from build123d import *

# Parameters (mm, degrees)
F0_R     = 10
F0_R_2   = 6
F1_DEPTH = 4
F0_R_3   = 2.6
F2_DEPTH = 4.5
F3_DEPTH = 10.5
F4_R     = 8.5
F5_DEPTH = 1.5
F7_R     = 1
F8_DEPTH = 0.2


# Not quite as in the source:
# - a fillet or chamfer that OpenCascade refuses, or shapes differently, is made with other operations: its cross-section is extruded or revolved along the edge and cut away or added


with BuildPart() as f1:
    # F0 (on Top) → F1 (new body)
    with BuildSketch(Plane.XY):
        with Locations((-11.3181825727, 20.5227266997)):
            Circle(F0_R)
        with Locations((-11.3181825727, 20.5227266997)):
            Circle(F0_R_2, mode=Mode.SUBTRACT)
    extrude(amount=F1_DEPTH)

    # F0 (on Top) → F2 (join)
    with BuildSketch(Plane.XY):
        with Locations((-11.3181825727, 20.5227266997)):
            Circle(F0_R_2)
        with Locations((-11.3181825727, 20.5227266997)):
            Circle(F0_R_3, mode=Mode.SUBTRACT)
    extrude(amount=F2_DEPTH)

    # F0 (on Top) → F3 (join)
    with BuildSketch(Plane.XY):
        with Locations((-11.3181825727, 20.5227266997)):
            Circle(F0_R_3)
    extrude(amount=F3_DEPTH)

    # F4 (on face) → F5 (cut)
    with BuildSketch(Plane(origin=(0, 0, 0), x_dir=(1, 0, 0), z_dir=(0, 0, -1))):
        with Locations((-11.3181825727, -20.5227266997)):
            Circle(F4_R)
    extrude(amount=-F5_DEPTH, mode=Mode.SUBTRACT)

    # F6: fillet of radius 20 on 1 edges, made by hand

    # F6_s1 → F6_t2 (revolve)
    with BuildSketch(Plane.XZ.offset(-20.5227266997)):
        with BuildLine():
            ThreePointArc((-2.8181825727, 0), (-6.5445413033, 1.1214168703), (-10.4175246495, 1.5))
            Line((-10.4175246495, 1.5), (-2.8181825727, 1.5))
            Line((-2.8181825727, 1.5), (-2.8181825727, 0))
        make_face()
    revolve(axis=Axis((-11.3181825727, 20.5227266997, 1.5), (0, 0, -1)))

    # F7
    f7_edges = [f1.edges().sort_by_distance(p)[0] for p in [
        (-21.318183, 20.522727, 0),
    ]]
    fillet(f7_edges, radius=F7_R)

    # F8 (cut): a face of the model
    f8_faces = [f1.faces().sort_by_distance(p)[0] for p in [
        (-21.0353398602, 20.5227266997, 4),
    ]]
    extrude(f8_faces, amount=-F8_DEPTH, mode=Mode.SUBTRACT)


solid = f1.part
Source: CAD feature listing. Evaluate the final solid. Frame: model axes, mm. A direction names the side the tool comes from. Give positions to 0.01 mm unless a question says otherwise; leave off trailing zeros. Order: outer loops, then holes, each group sorted by start corner. A loop starts at its lowest first (then second) coordinate and runs counter-clockwise, first axis right, second up. Notation, with made-up numbers: (72.25, -8) -> (78.25, -8) arc R23 cw to (78.25, 6) -> close; hole circle Ø5 at (-19.75, 60). An arc over 180 degrees is marked (long way). Write item = value, one per line.
Item 1: Ray query, probe 1 along Z at (x, y) = (-2.75, 21); probe 2 along Y at (x, z) = (-11.75, 5.75); probe 3 along Z at (x, y) = (-6.25, 17). Return the intervals inside material, ascending.
Check result:
probe_1 = 0 to 3.8
probe_2 = 17.96 to 23.09
probe_3 = 0.79 to 3.8
Item 2: Section query A-A (z = 2.5). Output: boundary loops of the cut face in (x, y), then the cut area to 3 significant figures.
Check result:
outline = circle Ø20 at (-11.32, 20.52)
area = 314 mm²
Item 3: Set-up query: faces 4 (the face through (-1.78, 23.53, 2.38)), 5 (the face through (-10, 18, 4.5)). Return all of +Z, -Z, +X, -X, +Y, -Y with unobstructed straight access to the full face (end or side cutting, diameter ignored); none if empty.
Check result:
face_4 = +Z, -Z
face_5 = +Z
Item 4: Contact query for flat-ended pins moving along their axis: pin 1 (4 mm diameter, centred on y = 17, z = 3, fed in from +X); pin 2 (8 mm diameter, centred on x = -15.5, y = 19, fed in from -Z); pin 3 (1.5 mm diameter, centred on y = 18.5, z = 2, fed in from -X). Output: stop coordinate, or through.
Check result:
pin_1 = -1.43
pin_2 = 0.02
pin_3 = -21.24
Item 5: Mould query, pull axis X, two halves, no side actions, for faces 1 (the face through (-11, 21, 1.5)), 2 (the face through (-8.916, 19.527, 7.458)), 3 (the face through (-11, 21, 10.5)). Classes: +X half, -X half, draft (parallel to the pull), parting line (faces both ways), or undercut.
Check result:
face_1 = undercut
face_2 = parting line
face_3 = draft
Item 6: Section query B-B (z = 7.25). Output: boundary loops of the cut face in (x, y), then the cut area to 3 significant figures.
Check result:
outline = circle Ø5.2 at (-11.32, 20.52)
area = 21.2 mm²
